from build123d import *
from build123d.topology import SkipClean

# Parameters (mm, degrees)
EXTRUDE_1_DEPTH      = 20
FILLET_1_R           = 10
FILLET_2_R           = 10
SKETCH_3_R           = 15
CUT_EXTRUDE_1_DEPTH  = 20
EXTRUDE_2_DEPTH      = 21
EXTRUDE_2_DEPTH_BACK = 1
SKETCH_2_R           = 40
CUT_EXTRUDE_2_DEPTH  = 15
SKETCH_5_R           = 30
EXTRUDE_3_DEPTH      = 15
SKETCH_5_3_R         = 15
SKETCH_5_3_R_2       = 10
EXTRUDE_4_DEPTH      = 10


with BuildPart() as part:
    # Sketch 1 → Extrude 1 (new body)
    with BuildSketch(Plane(origin=(0, 0, 0), x_dir=(1, 0, 0), z_dir=(0, 1, 0))):
        with BuildLine():
            ThreePointArc((43.301270189, 25), (0, 50), (-43.301270189, 25))
            Line((-43.301270189, 25), (43.301270189, 25))
        make_face()
        with BuildLine():
            ThreePointArc((-43.301270189, 25), (-50, 0), (-43.301270189, -25))
            Line((-43.301270189, -25), (43.301270189, -25))
            ThreePointArc((43.301270189, -25), (48.296291314, -12.940952255), (50, 0))
            ThreePointArc((50, 0), (48.296291314, 12.940952255), (43.301270189, 25))
            Line((43.301270189, 25), (-43.301270189, 25))
        make_face()
        with BuildLine():
            Line((43.301270189, -25), (-43.301270189, -25))
            ThreePointArc((-43.301270189, -25), (0, -50), (43.301270189, -25))
        make_face()
        with BuildLine():
            ThreePointArc((50, 0), (48.296291314, -12.940952255), (43.301270189, -25))
            Line((43.301270189, -25), (100, -25))
            Line((100, -25), (100, 25))
            Line((100, 25), (43.301270189, 25))
            ThreePointArc((43.301270189, 25), (48.296291314, 12.940952255), (50, 0))
        make_face()
        with BuildLine():
            Line((-100, 25), (-100, -25))
            Line((-100, -25), (-43.301270189, -25))
            ThreePointArc((-43.301270189, -25), (-50, 0), (-43.301270189, 25))
            Line((-43.301270189, 25), (-100, 25))
        make_face()
    extrude(amount=EXTRUDE_1_DEPTH)

    # Fillet 1
    fillet_1_edges = [part.edges().sort_by_distance(p)[0] for p in [
        (-43.301270189, 10, 25),
    ]]
    fillet(fillet_1_edges, radius=FILLET_1_R)

    # Fillet 2
    fillet_2_edges = [part.edges().sort_by_distance(p)[0] for p in [
        (43.301270189, 10, -25),
        (43.301270189, 10, 25),
        (-43.301270189, 10, -25),
    ]]
    fillet(fillet_2_edges, radius=FILLET_2_R)

    # Sketch 3 → Cut-Extrude 1 (cut)
    with BuildSketch(Plane(origin=(0, 0, 0), x_dir=(1, 0, 0), z_dir=(0, 1, 0))):
        with Locations((-100, 0)):
            Circle(SKETCH_3_R)
        with Locations((100, 0)):
            Circle(SKETCH_3_R)
    extrude(amount=CUT_EXTRUDE_1_DEPTH, mode=Mode.SUBTRACT)

    # Sketch 4 → Extrude 2 (add, two sides: drawn at the far end of the back side and taken through both)
    with BuildSketch(Plane(origin=(0, 0, 0), x_dir=(1, 0, 0), z_dir=(0, 1, 0)).offset(-EXTRUDE_2_DEPTH_BACK)):
        with BuildLine():
            ThreePointArc((-84, 0), (-88.686291501, 11.313708499), (-100, 16))
            Line((-100, 16), (-100, 15))
            ThreePointArc((-100, 15), (-89.393398282, 10.606601718), (-85, 0))
            ThreePointArc((-85, 0), (-89.393398282, -10.606601718), (-100, -15))
            Line((-100, -15), (-100, -16))
            ThreePointArc((-100, -16), (-88.686291501, -11.313708499), (-84, 0))
        make_face()
        with BuildLine():
            Line((100, -16), (100, -15))
            ThreePointArc((100, -15), (85, 0), (100, 15))
            Line((100, 15), (100, 16))
            ThreePointArc((100, 16), (84, 0), (100, -16))
        make_face()
    extrude(amount=EXTRUDE_2_DEPTH + EXTRUDE_2_DEPTH_BACK)

    # Sketch 2 → Cut-Extrude 2 (cut)
    with SkipClean():  # the faces are left unmerged after this step: merging them gives an invalid solid
        with BuildSketch(Plane(origin=(0, 0, 0), x_dir=(1, 0, 0), z_dir=(0, 1, 0))):
            with Locations(Location((0, 0, 0), (0, 0, 270))):
                Circle(SKETCH_2_R)
        extrude(amount=CUT_EXTRUDE_2_DEPTH, mode=Mode.SUBTRACT)

    # Sketch 5 → Extrude 3 (add)
    with SkipClean():  # the faces are left unmerged after this step: merging them gives an invalid solid
        with BuildSketch(Plane(origin=(0, 0, 0), x_dir=(1, 0, 0), z_dir=(0, 1, 0))):
            with Locations(Location((0, 0, 0), (0, 0, 270))):
                Circle(SKETCH_5_R)
        extrude(amount=EXTRUDE_3_DEPTH)

    # Sketch 5_3 → Extrude 4 (add)
    with SkipClean():  # the faces are left unmerged after this step: merging them gives an invalid solid
        with BuildSketch(Plane(origin=(0, 0, 0), x_dir=(1, 0, 0), z_dir=(0, 1, 0))):
            with Locations(Location((0, 0, 0), (0, 0, 270))):
                Circle(SKETCH_5_3_R)
            with Locations(Location((0, 0, 0), (0, 0, 270))):
                Circle(SKETCH_5_3_R_2, mode=Mode.SUBTRACT)
        extrude(amount=-EXTRUDE_4_DEPTH)


solid = part.part
Build history of the part. All positions in model axes, mm. A direction names the side the tool comes from. Round coordinates to 2 decimals unless told otherwise and drop trailing zeros. Write each loop counter-clockwise with the first axis right and the second up, starting at its lowest first coordinate (ties: lowest second). Pieces come first, ordered by that corner, then holes. Notation, with made-up numbers: M -14.5,48.25 L -0.5,48.25 A21 ccw -0.5,54.25 Z; hole C 10.25,-3.75 d6. An arc over 180 degrees is marked long. Answer as a JSON object with one key per item and string values. Group by question number.
(1) Cut at D-D (z = -18). Give the cut face in (x, y), and give its area (3 significant figures).
(2) Mould opens along Z. For faces 3 (the cylindrical face through (1.32, 7.4, -29.97)), 4 (the flat face through (-84.9, -1, -1.3)), 5 (the cylindrical face through (84.004, 20.493, -0.352)) say: pulls with the +Z half, pulls with the -Z half, needs draft (parallel to the pull), parting line crosses it, or undercut.
(3) Cut at A-A (y = -7). Give the cut face in (x, z).
(4) Which spindle directions (+Z, -Z, +X, -X, +Y, -Y) get a long thin tool onto all of the face, cutting with end or side? Do faces 1 (the cylindrical face through (0.664, 9.86, -49.996)), 2 (the flat face through (43, 0, -1)). Say none if no direction does.
(5) Drill centre lines: L1, parallel to X at y = 10, z = 0; L2, parallel to X at y = 4.5, z = -5.5; L3, parallel to Y at x = 65, z = 15. Where is each one in solid material? Low to high.
(6) Cut at C-C (z = 13). Give the cut face in (x, y).
(7) Cut at B-B (x = 0). Give the cut face in (y, z).
(8) Flat gauge pins, fed straight in: pin 1 (16 mm diameter, centred on x = 0, z = 0, fed in from -Y); pin 2 (16 mm diameter, centred on x = -71, y = 6, fed in from -Z); pin 3 (1.5 mm diameter, centred on y = 6.5, z = -11, fed in from +X); pin 4 (5 mm diameter, centred on x = 92, z = -8, fed in from -Y). Where does each tip first touch, or does it go through?
Responses:
{
 "1": {"outline": "M -100,0 L -35.72,0 L -35.72,15 L -24,15 L -24,0 L 24,0 L 24,15 L 35.72,15 L 35.72,0 L 100,0 L 100,20 L -100,20 Z", "area": "3,650 mm2"},
 "2": {"face 3": "undercut", "face 4": "needs draft", "face 5": "parting line crosses it"},
 "3": {"outline": "C 0,0 d30; hole C 0,0 d20"},
 "4": {"face 1": "-Z, +Y, -Y", "face 2": "-Y"},
 "5": {"L1": "x = -85 to -40, -30 to 30, 40 to 85", "L2": "x = -86.04 to -39.62, -29.49 to 29.49, 39.62 to 86.04", "L3": "y = 0 to 20"},
 "6": {"outline": "M -92.52,-1 L -90.67,-1 L -90.67,0 L -37.83,0 L -37.83,15 L -27.04,15 L -27.04,0 L -7.48,0 L -7.48,-10 L 7.48,-10 L 7.48,0 L 27.04,0 L 27.04,15 L 37.83,15 L 37.83,0 L 90.67,0 L 90.67,-1 L 92.52,-1 L 92.52,21 L 90.67,21 L 90.67,20 L -90.67,20 L -90.67,21 L -92.52,21 Z"},
 "7": {"outline": "M -10,-15 L 0,-15 L 0,-30 L 15,-30 L 15,-40 L 0,-40 L 0,-50 L 20,-50 L 20,50 L 0,50 L 0,40 L 15,40 L 15,30 L 0,30 L 0,15 L -10,15 L -10,10 L 0,10 L 0,-10 L -10,-10 Z"},
 "8": {"pin 1": "stops at y = 0", "pin 2": "stops at z = -25", "pin 3": "stops at x = 90.68", "pin 4": "passes through"}
}
